```python
from build123d import *

# Parameters (mm, degrees)
SKETCH_1_R                   = 45
SKETCH_1_R_2                 = 39
EXTRUDE_1_DEPTH              = 3.975
SKETCH_2_R                   = 47.5
SKETCH_2_R_2                 = 39
EXTRUDE_2_DEPTH              = 1.5
HOLE_WIZARD_M3_1_D           = 2.5
HOLE_WIZARD_M3_1_CSINK_D     = 3.05
HOLE_WIZARD_M3_1_CSINK_ANGLE = 90
PATTERN_CIRCULAR_1_COUNT     = 6
CHAMFER_1_SIZE               = 0.5


with BuildPart() as part:
    # 草图1 → 凸台-拉伸1 (new, symmetric)
    with BuildSketch(Plane(origin=(0, 0, 0), x_dir=(1, 0, 0), z_dir=(0, 1, 0))):
        with Locations(Location((0, 0, 0), (0, 0, 270))):
            Circle(SKETCH_1_R)
        with Locations(Location((0, 0, 0), (0, 0, 270))):
            Circle(SKETCH_1_R_2, mode=Mode.SUBTRACT)
    extrude(amount=EXTRUDE_1_DEPTH, both=True)

    # 草图2 → 凸台-拉伸2 (add)
    with BuildSketch(Plane(origin=(0, 3.975, 0), x_dir=(1, 0, 0), z_dir=(0, 1, 0))):
        with Locations(Location((0, 0, 0), (0, 0, 270))):
            Circle(SKETCH_2_R)
        with Locations(Location((0, 0, 0), (0, 0, 270))):
            Circle(SKETCH_2_R_2, mode=Mode.SUBTRACT)
    extrude(amount=EXTRUDE_2_DEPTH)

    # M3 螺纹孔1 (through all)
    with Locations(Plane(origin=(0, -3.975, 0), x_dir=(-1, 0, 0), z_dir=(0, -1, 0))):
        with Locations((0, 42)):
            hole_wizard_m3_1 = CounterSinkHole(HOLE_WIZARD_M3_1_D / 2, HOLE_WIZARD_M3_1_CSINK_D / 2, counter_sink_angle=HOLE_WIZARD_M3_1_CSINK_ANGLE)

    # 阵列(圆周)1: M3 螺纹孔1 ×6 about axis
    pattern_circular_1_axis = Axis((0, 0, 0), (0, 1, 0))
    for i in range(1, PATTERN_CIRCULAR_1_COUNT):
        add(hole_wizard_m3_1.rotate(pattern_circular_1_axis, i * 360 / PATTERN_CIRCULAR_1_COUNT), mode=Mode.SUBTRACT)

    # 倒角1
    chamfer_1_edges = [part.edges().sort_by_distance(p)[0] for p in [
        (0, -3.975, -45),
    ]]
    chamfer(chamfer_1_edges, length=CHAMFER_1_SIZE)


solid = part.part
```
Can you work these out from the model? Positions are in its coordinate system, mm. A direction names the side the tool comes from. Coordinates: 2 decimals unless noted, no trailing zeros. Write each loop counter-clockwise with the first axis right and the second up, starting at its lowest first coordinate (ties: lowest second). Pieces come first, ordered by that corner, then holes. Notation, with made-up numbers: M 28,47 L 44,47 A12 ccw 44,60 Z; hole C 46,38 d4. An arc over 180 degrees is marked long. Write item = value, one per line. Start each with the question number.
Q1. If we section it at B-B, the plane y = 2: Write out the boundary of the cut face in (x, z), then the cut area to 3 significant figures.
Q2. Thinking about a two-plate mould opening in X: for faces 1 (the face through (0.16, 0.95, 43.24)), 2 (the face through (-17.235, 0.302, 41.569)), 3 (the face through (39, 5.475, -4)), which applies, released by +X, released by -X, zero draft, split by the parting line, or undercut?
Q3. If we section it at A-A, the plane x = 0: Write out the boundary of the cut face in (y, z) (3 decimals), then the cut area to 3 significant figures.
Q4. If I drill on L1, parallel to X at y = 1, z = -21; L2, parallel to X at y = -1, z = 0; L3, parallel to Z at x = -0.5, y = 0.5, over which ranges is the centre line in solid material (lowest first)? Write a range as [from, to].
Q5. On a 3-axis mill with a long thin cutter (end or side, diameter ignored), from which of +Z, -Z, +X, -X, +Y, -Y can I reach the whole of each face in a straight line? I mean faces 4 (the face through (36.95, 0.95, 22.11)), 5 (the face through (-42, 3.975, 17)). Say none if no direction works.
Q6. If we section it at C-C, the plane z = 21: State how many separate pieces and enclosed holes the cut face has, then the cut area to 3 significant figures.
Q7. I'm going to push flat-ended pins straight in: pin 1 (5 mm diameter, centred on y = -1.5, z = -36, fed in from +X); pin 2 (1.5 mm diameter, centred on x = -12, y = 0, fed in from +Z). Where does each tip first touch, or does it pass through?
Check sheet entries:
q1.outline = C 0,0 d90; hole C 0,0 d78; hole C -36.37,-21 d2.5; hole C -36.37,21 d2.5; hole C 0,-42 d2.5; hole C 0,42 d2.5; hole C 36.37,-21 d2.5; hole C 36.37,21 d2.5
q1.area = 1,550 mm²
q2.face_1 = undercut
q2.face_2 = split by the parting line
q2.face_3 = zero draft
q3.outline = M -3.975,-44.5 L -3.475,-45 L 3.975,-45 L 3.975,-47.5 L 5.475,-47.5 L 5.475,-43.25 L -3.7,-43.25 L -3.975,-43.525 Z; M -3.975,-40.475 L -3.7,-40.75 L 5.475,-40.75 L 5.475,-39 L -3.975,-39 Z; M -3.975,39 L 5.475,39 L 5.475,40.75 L -3.7,40.75 L -3.975,40.475 Z; M -3.975,43.525 L -3.7,43.25 L 5.475,43.25 L 5.475,47.5 L 3.975,47.5 L 3.975,45 L -3.475,45 L -3.975,44.5 Z
q3.area = 73.2 mm²
q4.L1 = [-39.8, -37.62], [-35.12, -32.86], [32.86, 35.12], [37.62, 39.8]
q4.L2 = [-45, -39], [39, 45]
q4.L3 = [-45, -43.15], [-40.85, -39], [39, 40.85], [43.15, 45]
q5.face_4 = +Y, -Y
q5.face_5 = -Y
q6.separate_pieces = 4
q6.enclosed_holes = 0
q6.area = 91.8 mm²
q7.pin_1 = 30.05
q7.pin_2 = 43.57
